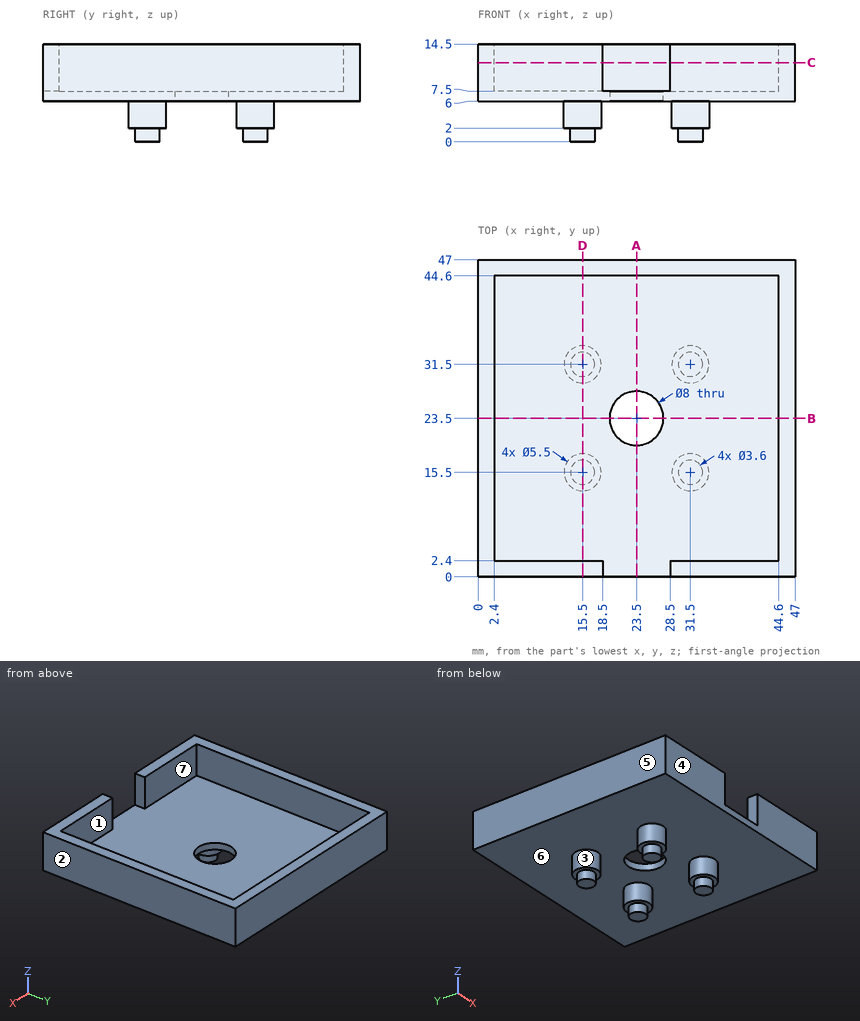
Study the drawing (mm; zero at the part's minimum x, y, z) and answer. A direction names the side the tool comes from. Give positions to 0.01 mm unless a question says otherwise; leave off trailing zeros. Loops run counter-clockwise (first coordinate to the right, second up) from the corner with the lowest first, then second, coordinate; pieces in that order, holes last. Notation, with made-up numbers: M -14.5,-3.5 L -9.5,-3.5 A26 cw -9.5,31.5 Z; hole C 34,64.25 d8. An arc over 180 degrees is marked long. One line per item, written item: value. Start each with the question number.
1. Each of these flat-tipped pins is pushed along its axis until it touches: P1, Ø12, axis at x = 15.5, y = 20, coming from the +Z side; P2, Ø2, axis at x = 11, y = 10, coming from the -Z side. Where does it stop, or does it pass through?
2. Find section C-C (z = 11.75). Give the vertices of the cut face in (x, y), and give its area (3 significant figures).
3. Find the intervals of material crossed by probe 1 along Y at (x, z) = (23.5, 6.5); probe 2 along X at (y, z) = (44.5, 14.25), in increasing order.
4. Which of the six approach directions +Z, -Z, +X, -X, +Y, -Y give full straight-line access (tool end or side, diameter ignored) to the marked faces 5, 6 and 7?
5. Find section B-B (y = 23.5). Give the vertices of the cut face in (x, z), and give its area (3 significant figures).
6. Find section A-A (x = 23.5). Give the vertices of the cut face in (y, z).
7. Determine the mould class of the marked faces 1, 2, 3 and 4 for opening direction X: released by +X, released by -X, zero draft, split by the parting line, or undercut.
8. Find section D-D (x = 15.5). Give the vertices of the cut face in (y, z).
Reported:
1. P1: stops at z = 7.5
1. P2: stops at z = 6
2. outline: M 0,0 L 18.5,0 L 18.5,2.4 L 2.4,2.4 L 2.4,44.6 L 44.6,44.6 L 44.6,2.4 L 28.5,2.4 L 28.5,0 L 47,0 L 47,47 L 0,47 Z
2. area: 404 mm²
3. probe 1: y = 0 to 19.5, 27.5 to 47
3. probe 2: x = 0 to 2.4, 44.6 to 47
4. face 5: +Z, -Z, -X, +Y, -Y
4. face 6: -Z
4. face 7: +Z
5. outline: M 0,6 L 19.5,6 L 19.5,7.5 L 2.4,7.5 L 2.4,14.5 L 0,14.5 Z; M 27.5,6 L 47,6 L 47,14.5 L 44.6,14.5 L 44.6,7.5 L 27.5,7.5 Z
5. area: 92.1 mm²
6. outline: M 0,6 L 19.5,6 L 19.5,7.5 L 0,7.5 Z; M 27.5,6 L 47,6 L 47,14.5 L 44.6,14.5 L 44.6,7.5 L 27.5,7.5 Z
7. face 1: undercut
7. face 2: released by +X
7. face 3: undercut
7. face 4: zero draft
8. outline: M 0,6 L 12.75,6 L 12.75,2 L 13.7,2 L 13.7,0 L 17.3,0 L 17.3,2 L 18.25,2 L 18.25,6 L 28.75,6 L 28.75,2 L 29.7,2 L 29.7,0 L 33.3,0 L 33.3,2 L 34.25,2 L 34.25,6 L 47,6 L 47,14.5 L 44.6,14.5 L 44.6,7.5 L 2.4,7.5 L 2.4,14.5 L 0,14.5 Z
